The listing builds one solid part. Answer for the finished solid, in the listing's coordinates (mm). A direction names the side the tool comes from. Give positions to 0.01 mm unless a question says otherwise; leave off trailing zeros. Order: outer loops, then holes, each group sorted by start corner. A loop starts at its lowest first (then second) coordinate and runs counter-clockwise, first axis right, second up. Notation, with made-up numbers: (60.5, -9.5) - (84.5, -9.5) arc R16 ccw to (84.5, 5.5) - close; hole circle Ø4 at (49, -34). An arc over 180 degrees is marked (long way). Answer in a Markdown table with one row per item.
from build123d import *

# Parameters (mm, degrees)
EXTRU_MINCE1_DEPTH      = 9.5
ESQUISSE2_R             = 1.6
ENL_V_MAT_EXTRU_1_DEPTH = 27.196373795
ENL_V_START             = -2.5
ESQUISSE4_R             = 3
ENL_V_MAT_EXTRU_3_DEPTH = 24.696373795
SKETCH2_W               = 19
SKETCH2_H               = 8
CUT_EXTRUDE2_DEPTH      = 22.960191256
SKETCH4_W               = 19
SKETCH4_H               = 2
BOSS_EXTRUDE2_DEPTH     = 3
BOSS_EXTRUDE3_DEPTH     = 10
SKETCH6_R               = 1.5
CUT_EXTRUDE3_DEPTH      = 29.570089254
CUT_EXTRUDE6_DEPTH      = 29.570089254
LPATTERN1_COUNT         = 2
LPATTERN1_PITCH         = 8


with BuildPart() as part:
    # Esquisse1 → Extru.-Mince1 (new, symmetric)
    with BuildSketch(Plane(origin=(0, 0, 0), x_dir=(0, 0, -1), z_dir=(1, 0, 0))):
        Polygon((20, 0), (0, 0), (0, -14), (6, -14), (6, -6), (20, -6), align=None)
    extrude(amount=EXTRU_MINCE1_DEPTH, both=True)

    # Esquisse2 → Enl_v. mat.-Extru.1 (cut, through all)
    with BuildSketch(Plane(origin=(0, 0, 0), x_dir=(1, 0, 0), z_dir=(0, 1, 0))):
        with Locations(Location((0, 14, 0), (0, 0, 90))):
            Circle(ESQUISSE2_R)
    enl_v_mat_extru_1 = extrude(amount=-ENL_V_MAT_EXTRU_1_DEPTH, mode=Mode.SUBTRACT)

    # Esquisse4 → Enl_v. mat.-Extru.3 (cut, through all)
    with BuildSketch(Plane(origin=(0, 0, 0), x_dir=(1, 0, 0), z_dir=(0, 1, 0)).offset(ENL_V_START)):
        with Locations(Location((0, 14, 0), (0, 0, 270))):
            Circle(ESQUISSE4_R)
    enl_v_mat_extru_3 = extrude(amount=-ENL_V_MAT_EXTRU_3_DEPTH, mode=Mode.SUBTRACT)

    # Sketch2 → Cut-Extrude2 (cut, through all)
    with BuildSketch(Plane(origin=(0, 0, -6), x_dir=(-1, 0, 0), z_dir=(0, 0, -1))):
        with Locations((0, -10)):
            Rectangle(SKETCH2_W, SKETCH2_H)
    extrude(amount=-CUT_EXTRUDE2_DEPTH, mode=Mode.SUBTRACT)

    # Sketch4 → Boss-Extrude2 (add)
    with BuildSketch(Plane.XZ.offset(6)):
        with Locations((0, -1)):
            Rectangle(SKETCH4_W, SKETCH4_H)
        with Locations((0, -19)):
            Rectangle(SKETCH4_W, SKETCH4_H)
    extrude(amount=BOSS_EXTRUDE2_DEPTH)

    # Sketch5 → Boss-Extrude3 (add)
    with BuildSketch(Plane(origin=(9.5, 0, 0), x_dir=(0, 0, -1), z_dir=(1, 0, 0))):
        Polygon((0, 0), (0, -9), (2, -9), (2, -6), (18, -6), (18, -9), (20, -9), (20, 0), align=None)
    extrude(amount=BOSS_EXTRUDE3_DEPTH)

    # Sketch6 → Cut-Extrude3 (cut, through all)
    with BuildSketch(Plane.XZ.offset(6)):
        with Locations(Location((11.05, -6.15, 0), (0, 0, 270))):
            Circle(SKETCH6_R)
    extrude(amount=-CUT_EXTRUDE3_DEPTH, mode=Mode.SUBTRACT)

    # Sketch7 → Cut-Extrude6 (cut, through all)
    with BuildSketch(Plane.XZ.offset(6)):
        with BuildLine():
            Line((11.05, -4.65), (15.450055752, -4.65))
            ThreePointArc((15.450055752, -4.65), (16.950055752, -6.15), (15.450055752, -7.65))
            Line((15.450055752, -7.65), (11.05, -7.65))
            ThreePointArc((11.05, -7.65), (12.55, -6.15), (11.05, -4.65))
        make_face()
    extrude(amount=-CUT_EXTRUDE6_DEPTH, mode=Mode.SUBTRACT)

    # LPattern1: Enl_v. mat.-Extru.1, Enl_v. mat.-Extru.3 ×2
    with Locations(*[(0, 0, i * LPATTERN1_PITCH) for i in range(1, LPATTERN1_COUNT)]):
        add(enl_v_mat_extru_1, mode=Mode.SUBTRACT)
        add(enl_v_mat_extru_3, mode=Mode.SUBTRACT)


solid = part.part
Item 1: Which of the six approach directions +Z, -Z, +X, -X, +Y, -Y give full straight-line access (tool end or side, diameter ignored) to faces 1 (the face through (5, -7, -18)), 2 (the face through (19.5, -3, -10)), 3 (the face through (5, -9, -19)), 4 (the face through (16.95, -3.04, -6.12)), 5 (the face through (-1.3, -2.5, -12.7))?
Answer block:
| item | result |
|---|---|
| face 1 | +X, -X, -Y |
| face 2 | +Z, -Z, +X, +Y, -Y |
| face 3 | +Z, -Z, +X, -X, -Y |
| face 4 | +Y, -Y |
| face 5 | -Y |
Item 2: Find section D-D on x = 8. Write down the section's boundary in (y, z), then the cut area to 3 significant figures.
Answer block:
| item | result |
|---|---|
| outline | (-9, -20) - (0, -20) - (0, 0) - (-9, 0) - (-9, -2) - (-6, -2) - (-6, -18) - (-9, -18) - close |
| area | 132 mm² |
Item 3: Determine the mould class of faces 6 (the face through (0, -4, -17)), 7 (the face through (5, -9, -1)), 8 (the face through (5, -4, 0)) for opening direction Z: pulls with the +Z half, pulls with the -Z half, needs draft (parallel to the pull), parting line crosses it, or undercut.
Answer block:
| item | result |
|---|---|
| face 6 | undercut |
| face 7 | needs draft |
| face 8 | pulls with the +Z half |
Item 4: Find section C-C on x = 13.75. Write down the section's boundary in (y, z), then the cut area to 3 significant figures.
Answer block:
| item | result |
|---|---|
| outline | (-9, -20) - (0, -20) - (0, -7.65) - (-6, -7.65) - (-6, -18) - (-9, -18) - close; (-9, -2) - (-6, -2) - (-6, -4.65) - (0, -4.65) - (0, 0) - (-9, 0) - close |
| area | 114 mm² |
Item 5: Consider line 1 (Z direction, x = -4, y = -7); line 2 (X direction, y = -5, z = -14); line 3 (X direction, y = -4.45, z = -6). Determine where each line is inside the solid, lowest interval first.
Answer block:
| item | result |
|---|---|
| line 1 | -20 to -18, -2 to 0 |
| line 2 | -9.5 to -3, 3 to 19.5 |
| line 3 | -9.5 to -3, 3 to 9.56, 16.94 to 19.5 |
Item 6: Find section A-A on x = 0. Write down the section's boundary in (y, z), then the cut area to 3 significant figures.
Answer block:
| item | result |
|---|---|
| outline | (-9, -20) - (0, -20) - (0, -15.6) - (-2.5, -15.6) - (-2.5, -17) - (-6, -17) - (-6, -18) - (-9, -18) - close; (-9, -2) - (-6, -2) - (-6, -3) - (-2.5, -3) - (-2.5, -4.4) - (0, -4.4) - (0, 0) - (-9, 0) - close; (-6, -11) - (-2.5, -11) - (-2.5, -12.4) - (0, -12.4) - (0, -7.6) - (-2.5, -7.6) - (-2.5, -9) - (-6, -9) - close |
| area | 74.0 mm² |
Item 7: Find section B-B on z = -6.15. Write down the section's boundary in (x, y), then the cut area to 3 significant figures.
Answer block:
| item | result |
|---|---|
| outline | (-9.5, -6) - (-3, -6) - (-3, -2.5) - (-1.59, -2.5) - (-1.59, 0) - (-9.5, 0) - close; (1.59, -2.5) - (3, -2.5) - (3, -6) - (9.55, -6) - (9.55, 0) - (1.59, 0) - close; (16.95, -6) - (19.5, -6) - (19.5, 0) - (16.95, 0) - close |
| area | 101 mm² |
Item 8: Each of these flat-tipped pins is pushed along its axis until it touches: P1, Ø1.9, axis at x = 0, z = -6, coming from the +Y side; P2, Ø6.5, axis at x = -0.5, z = -6, coming from the -Y side; P3, Ø3, axis at x = -1, z = -15, coming from the -Y side. Where does it stop, or does it pass through?
Answer block:
| item | result |
|---|---|
| P1 | through |
| P2 | y = -6 |
| P3 | y = -2.5 |
